Could you check a few things on this model? Use its own coordinates, in mm. A direction names the side the tool comes from. Give positions to 0.01 mm unless a question says otherwise; leave off trailing zeros. Loops run counter-clockwise (first coordinate to the right, second up) from the corner with the lowest first, then second, coordinate; pieces in that order, holes last.
1. Thinking about a two-plate mould opening in Z: for faces 3 (the flat face through (38, 1, 7.5)), 4 (the flat face through (-11.911, 2, 3)), 5 (the cylindrical face through (36.003, 1.479, 2.483)), 6 (the cylindrical face through (-35.956, 1.479, 2.375)), which applies, +Z half, -Z half, draft (parallel to the pull), parting line (faces both ways), or undercut?
2. I need wall thicknesses on line 1 along X through (y, z) = (0.95, 5.25) (3 decimals); line 2 along X through (y, z) = (1, 3.5) (3 decimals); line 3 along X through (y, z) = (1.15, 1.75) (3 decimals). Which ranges of each line are inside material? Lowest first, please.
3. For faces 1 (the flat face through (-55.055, 1, 0)), 2 (the flat face through (4, 2, -2)), which set-ups out of +Z, -Z, +X, -X, +Y, -Y let a thin tool reach every point of the face, with its end or its side?
4. Imagine slicing it at B-B (x = 12). List the corners of the cut face in (y, z) for me, plus the area to 3 significant figures.
5. For P1, Ø2.5, axis at x = -49.94, z = -1.63, coming from the -Y side; P2, Ø0.9, axis at x = 10, y = 1, coming from the +Z side, each with a flat end and sliding along its axis, tell me the tip position at first contact or that it passes through.
6. Imagine slicing it at A-A (y = 1.05). List the corners of the cut face in (x, z) for me (3 decimals).
```python
from build123d import *

# Parameters (mm, degrees)
CROQUIS1_W              = 110.11
CROQUIS1_H              = 15
CROQUIS1_R              = 2.1
CROQUIS1_R_2            = 1.25
SALIENTE_EXTRUIR1_DEPTH = 3
CROQUIS4_W              = 30.354739951
CROQUIS4_H              = 9.499551224
CORTAR_EXTRUIR2_DEPTH   = 3
CROQUIS5_W              = 2.625048137
CROQUIS5_H              = 9.499551224
CORTAR_EXTRUIR3_DEPTH   = 3


with BuildPart() as part:
    # Croquis1 → Saliente-Extruir1 (new body)
    with BuildSketch(Plane(origin=(0, 0, 0), x_dir=(1, 0, 0), z_dir=(0, 1, 0))):
        Rectangle(CROQUIS1_W, CROQUIS1_H)
        with Locations(Location((50.055, 2.5, 0), (0, 0, 270))):
            Circle(CROQUIS1_R, mode=Mode.SUBTRACT)
        with Locations(Location((-49.941192306, 1.62734645, 0), (0, 0, 270))):
            Circle(CROQUIS1_R, mode=Mode.SUBTRACT)
        with Locations(Location((-20.765904609, -2.646032213, 0), (0, 0, 270))):
            Circle(CROQUIS1_R_2, mode=Mode.SUBTRACT)
        with Locations(Location((-34.735904609, -2.646032213, 0), (0, 0, 270))):
            Circle(CROQUIS1_R_2, mode=Mode.SUBTRACT)
        with Locations(Location((-15.735904609, -2.646032213, 0), (0, 0, 270))):
            Circle(CROQUIS1_R_2, mode=Mode.SUBTRACT)
        with Locations(Location((34.764095391, -2.646032213, 0), (0, 0, 270))):
            Circle(CROQUIS1_R_2, mode=Mode.SUBTRACT)
    extrude(amount=SALIENTE_EXTRUIR1_DEPTH)

    # Croquis4 → Cortar-Extruir2 (cut)
    with BuildSketch(Plane(origin=(0, 3, 0), x_dir=(1, 0, 0), z_dir=(0, 1, 0))):
        with Locations((3.265938607, -2.750224388)):
            Rectangle(CROQUIS4_W, CROQUIS4_H)
    extrude(amount=-CORTAR_EXTRUIR2_DEPTH, mode=Mode.SUBTRACT)

    # Croquis5 → Cortar-Extruir3 (cut)
    with BuildSketch(Plane(origin=(0, 3, 0), x_dir=(1, 0, 0), z_dir=(0, 1, 0))):
        with Locations((19.755832652, -2.750224388)):
            Rectangle(CROQUIS5_W, CROQUIS5_H)
    extrude(amount=-CORTAR_EXTRUIR3_DEPTH, mode=Mode.SUBTRACT)


solid = part.part
```
Derived:
1. face 3: +Z half
1. face 4: draft
1. face 5: undercut
1. face 6: undercut
2. line 1: x = -55.055 to -11.911, 21.068 to 55.055
2. line 2: x = -55.055 to -35.649, -33.823 to -21.679, -19.853 to -16.649, -14.823 to -11.911, 21.068 to 33.851, 35.677 to 55.055
2. line 3: x = -55.055 to -35.607, -33.864 to -21.637, -19.894 to -16.607, -14.864 to -11.911, 21.068 to 33.893, 35.636 to 55.055
3. face 1: +Z, -Z, -X, +Y, -Y
3. face 2: +Z, +Y, -Y
4. outline: (0, -7.5) - (3, -7.5) - (3, -2) - (0, -2) - close
4. area: 16.5 mm2
5. P1: passes through
5. P2: stops at z = -2
6. outline: (-55.055, -7.5) - (55.055, -7.5) - (55.055, 7.5) - (21.068, 7.5) - (21.068, -2) - (-11.911, -2) - (-11.911, 7.5) - (-55.055, 7.5) - close; hole circle Ø4.2 at (-49.941, -1.627); hole circle Ø2.5 at (-34.736, 2.646); hole circle Ø2.5 at (-20.766, 2.646); hole circle Ø2.5 at (-15.736, 2.646); hole circle Ø2.5 at (34.764, 2.646); hole circle Ø4.2 at (50.055, -2.5)
